Part model, mm, in its own coordinate system. Give positions to 0.01 mm unless a question says otherwise; leave off trailing zeros. Order: outer loops, then holes, each group sorted by start corner. A loop starts at its lowest first (then second) coordinate and runs counter-clockwise, first axis right, second up. Notation, with made-up numbers: M 13.25,78.5 L 55.25,78.5 A26 cw 55.25,100.5 Z; hole C 18.5,71.5 d10. An arc over 180 degrees is marked long. Write each question's results on one line, items separated by ' | '. Start each with the question number.
from build123d import *

# Parameters (mm, degrees)
BOSS_EXTRUDE1_DEPTH     = 250
SKETCH3_R               = 2.55
BOSS_EXTRUDE2_DEPTH     = 17.3825
SKETCH8_W               = 12.3825
SKETCH8_H               = 2
CUT_EXTRUDE4_DEPTH      = 251
SKETCH9_W               = 2
SKETCH9_H               = 12.3825
CUT_EXTRUDE5_DEPTH      = 1
SKETCH10_W              = 2.5
SKETCH10_H              = 4.00875
BOSS_EXTRUDE3_DEPTH     = 8.7625
SKETCH11_R              = 1.25
CUT_EXTRUDE6_DEPTH      = 247.638802
SKETCH14_W              = 3
SKETCH14_H              = 5
CUT_EXTRUDE7_DEPTH      = 4
SKETCH15_W              = 3.5
SKETCH15_H              = 4.7625
CUT_EXTRUDE9_DEPTH      = 1
MIRROR8_COPY_1_SKETCH_W = 3.5
MIRROR8_COPY_1_SKETCH_H = 4.7625
MIRROR8_COPY_1_DEPTH    = 1


with BuildPart() as part:
    # Sketch1 → Boss-Extrude1 (new body)
    with BuildSketch(Plane.YZ):
        Polygon((0, 4.7625), (-2.5, 4.7625), (-2.5, -4), (14.8825, -4), (14.8825, 4.7625), (12.3825, 4.7625), (12.3825, 0), (0, 0), align=None)
    extrude(amount=BOSS_EXTRUDE1_DEPTH)

    # Sketch3 → Boss-Extrude2 (add)
    with BuildSketch(Plane.XZ.offset(2.5)):
        with BuildLine():
            Line((120.019401026, -4), (129.980598974, -4))
            Line((129.980598974, -4), (129.980598974, -9))
            ThreePointArc((129.980598974, -9), (125.66141047, -15.191034327), (120.019401026, -10.175854887))
            Line((120.019401026, -10.175854887), (120.019401026, -4))
        make_face()
        with Locations((125.069401026, -10.175854887)):
            Circle(SKETCH3_R, mode=Mode.SUBTRACT)
    extrude(amount=-BOSS_EXTRUDE2_DEPTH)

    # Sketch8 → Cut-Extrude4 (cut, through all)
    with BuildSketch(Plane.YZ.offset(250)):
        with Locations((6.19125, -2)):
            Rectangle(SKETCH8_W, SKETCH8_H)
    extrude(amount=-CUT_EXTRUDE4_DEPTH, mode=Mode.SUBTRACT)

    # Sketch9 → Cut-Extrude5 (cut)
    with BuildSketch(Plane(origin=(0, 0, -4), x_dir=(-1, 0, 0), z_dir=(0, 0, -1))):
        with Locations((-117.519401026, 6.19125)):
            Rectangle(SKETCH9_W, SKETCH9_H)
    cut_extrude5 = extrude(amount=-CUT_EXTRUDE5_DEPTH, mode=Mode.SUBTRACT)

    # Mirror1: Cut-Extrude5 across plane
    add(cut_extrude5.mirror(Plane.ZY.offset(-125.069401026)), mode=Mode.SUBTRACT)

    # Sketch10 → Boss-Extrude3 (add)
    with BuildSketch(Plane.XY.offset(4.7625)):
        with Locations((1.25, 16.886875)):
            Rectangle(SKETCH10_W, SKETCH10_H)
        with Locations((1.25, -4.504375)):
            Rectangle(SKETCH10_W, SKETCH10_H)
    boss_extrude3 = extrude(amount=-BOSS_EXTRUDE3_DEPTH)

    # Mirror2: Boss-Extrude3 across plane
    add(boss_extrude3.mirror(Plane.ZY.offset(-125.069401026)))

    # Sketch11 → Cut-Extrude6 (cut)
    with BuildSketch(Plane.YZ.offset(250.138802052)):
        with Locations((16.35125, -1.46)):
            Circle(SKETCH11_R)
        with Locations((-3.96875, -1.46)):
            Circle(SKETCH11_R)
    cut_extrude6 = extrude(amount=-CUT_EXTRUDE6_DEPTH, mode=Mode.SUBTRACT)

    # Mirror3: Cut-Extrude6 across plane
    add(cut_extrude6.mirror(Plane.ZY.offset(-125.069401026)), mode=Mode.SUBTRACT)

    # Sketch14 → Cut-Extrude7 (cut)
    with BuildSketch(Plane.XY.offset(4.7625)):
        with Locations((1.5, -4.00875)):
            Rectangle(SKETCH14_W, SKETCH14_H)
        with Locations((1.5, 16.39125)):
            Rectangle(SKETCH14_W, SKETCH14_H)
    cut_extrude7 = extrude(amount=-CUT_EXTRUDE7_DEPTH, mode=Mode.SUBTRACT)

    # Mirror4: Cut-Extrude7 across plane
    add(cut_extrude7.mirror(Plane.ZY.offset(-125.069401026)), mode=Mode.SUBTRACT)

    # Sketch15 → Cut-Extrude9 (cut)
    with BuildSketch(Plane(origin=(0, -2.5, 0), x_dir=(-1, 0, 0), z_dir=(0, -1, 0))):
        with Locations((-4.25, 1.61875)):
            Rectangle(SKETCH15_W, SKETCH15_H)
    cut_extrude9 = extrude(amount=-CUT_EXTRUDE9_DEPTH, mode=Mode.SUBTRACT)

    # Mirror7: Cut-Extrude9 across plane
    add(cut_extrude9.mirror(Plane.ZX.offset(6.19125)), mode=Mode.SUBTRACT)

    # Mirror8: Cut-Extrude9 across plane
    add(cut_extrude9.mirror(Plane.ZY.offset(-125.069401026)), mode=Mode.SUBTRACT)

    # Mirror8 copy 1 sketch → Mirror8 copy 1 (cut)
    with BuildSketch(Plane(origin=(250.138802052, 14.8825, 0), x_dir=(1, 0, 0), z_dir=(0, 1, 0))):
        with Locations((-4.25, 1.61875)):
            Rectangle(MIRROR8_COPY_1_SKETCH_W, MIRROR8_COPY_1_SKETCH_H)
    extrude(amount=-MIRROR8_COPY_1_DEPTH, mode=Mode.SUBTRACT)


solid = part.part
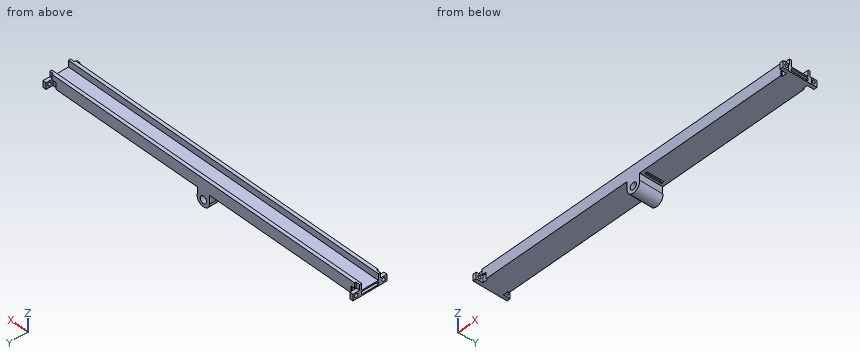
(1) Drop flat-ended pins along their axis: P1, Ø2, axis at y = -3, z = -12.5, coming from the +X side; P2, Ø0.9, axis at x = 248.5, z = 2, coming from the -Y side; P3, Ø1.5, axis at y = 3.5, z = -9.5, coming from the -X side; P4, Ø2.5, axis at y = -5, z = -1, coming from the +X side. Give the stop position or say it passes through.
(2) Saw through at B-B on x = 88. Give the cut face in (y, z).
(3) Probe L1, parallel to Y at x = 1.15, z = -1.46; L2, parallel to Z at x = 32.5, y = 1.75; L3, parallel to X at y = -4.5, z = -3. List the from-to ranges inside material, lowest first.
(4) Saw through at A-A on y = 9.5. Give the cut face in (x, z).
Taken from the geometry:
1) P1: stops at x = 129.9 | P2: stops at y = -1.51 | P3: stops at x = 120.02 | P4: stops at x = 250.14
2) outline: M -2.5,-4 L 14.88,-4 L 14.88,4.76 L 12.38,4.76 L 12.38,0 L 0,0 L 0,4.76 L -2.5,4.76 Z; hole M 0,-3 L 12.38,-3 L 12.38,-1 L 0,-1 Z
3) L1: y = -6.51 to -5.22, -2.72 to 0, 12.38 to 15.1, 17.6 to 18.89 | L2: z = -4 to -3, -1 to 0 | L3: x = 0 to 2.5, 247.64 to 250.14
4) outline: M 0,-4 L 116.52,-4 L 116.52,-3 L 0,-3 Z; M 0,-1 L 250,-1 L 250,0 L 0,0 Z; M 118.52,-4 L 120.02,-4 L 120.02,-10.18 A5.05 ccw long 129.98,-9 L 129.98,-4 L 131.62,-4 L 131.62,-3 L 118.52,-3 Z; M 133.62,-4 L 250,-4 L 250,-3 L 133.62,-3 Z; hole C 125.07,-10.18 d5.1
